Read the model definition and answer for the solid it produces. Units are mm, in the model's axes. A direction names the side the tool comes from. Coordinates: 2 decimals unless noted, no trailing zeros. Write each loop counter-clockwise with the first axis right and the second up, starting at its lowest first coordinate (ties: lowest second). Pieces come first, ordered by that corner, then holes.
Item 1: Section D-D (x = 66.04) is taken. Give the vertices of the cut face in (y, z), then the cut area to 3 significant figures.
Item 2: Section C-C (y = 1.5) is taken. State how many separate pieces and enclosed holes the cut face has, then the cut area to 3 significant figures.
Item 3: Section A-A (z = 0) is taken. Give the vertices of the cut face in (x, y) (3 decimals), then the cut area to 3 significant figures.
Item 4: Determine the mould class of faces 3 (the face through (-46.367, 3.131, -60.47)), 4 (the face through (1, 0, 33)), 5 (the face through (69.262, 3.219, 1.015)) for opening direction X: released by +X, released by -X, zero draft, split by the parting line, or undercut.
Item 5: Section B-B (x = 0) is taken. Give the vertices of the cut face in (y, z) (3 decimals).
Item 6: Straight lines are drawn through the part: probe 1 along X at (y, z) = (1, -0.5); probe 2 along X at (y, z) = (2.25, 3); probe 3 along Z at (x, y) = (46, 3.75). For each, find the intervals that lie inside material, in ascending order.
Item 7: Each of these flat-tipped pins is pushed along its axis until it touches: P1, Ø11, axis at x = 46.7, z = 46.7, coming from the +Y side; P2, Ø5.5, axis at x = 46.7, z = -46.7, coming from the -Y side; P3, Ø3, axis at x = -43.5, y = 3, coming from the +Z side; P4, Ø2, axis at y = 4, z = 37, coming from the -X side. Where does it stop, or does it pass through?
Item 8: A tool of negligible diameter and unlimited length cuts with its end or side. For faces 1 (the face through (48.755, 3.219, -44.018)), 2 (the face through (-34.094, 4.114, -7.571)), from which of +Z, -Z, +X, -X, +Y, -Y can it reach the whole face along a straight path? Write none if from no direction.
from build123d import *

# Parameters (mm, degrees)
SKETCH1_R           = 76.2
SKETCH1_R_2         = 34.925
BOSS_EXTRUDE1_DEPTH = 6.35
CIRPATTERN1_COUNT   = 8
CHAMFER1_SIZE       = 1.27
SKETCH6_R           = 34.925
SKETCH6_R_2         = 31.75
BOSS_EXTRUDE2_DEPTH = 3.175


with BuildPart() as part:
    # Sketch1 → Boss-Extrude1 (new body)
    with BuildSketch(Plane(origin=(0, 0, 0), x_dir=(1, 0, 0), z_dir=(0, 1, 0))):
        with Locations(Location((0, 0, 0), (0, 0, 270))):
            Circle(SKETCH1_R)
        with Locations(Location((0, 0, 0), (0, 0, 270))):
            Circle(SKETCH1_R_2, mode=Mode.SUBTRACT)
    extrude(amount=BOSS_EXTRUDE1_DEPTH)

    # Sketch4 → 1_4 Clearance Hole1 (revolve, cut)
    with BuildSketch(Plane(origin=(0, 6.35, 66.04), x_dir=(0, 0, 1), z_dir=(1, 0, 0))):
        Polygon((0, 0), (0, 27.429827343), (3.3782, 25.4), (3.3782, 0), align=None)
    f_1_4_clearance_hole1 = revolve(axis=Axis((0, 12.7, 66.04), (0, -1, 0)), mode=Mode.SUBTRACT)

    # CirPattern1: 1_4 Clearance Hole1 ×8 about axis
    cirpattern1_axis = Axis((0, 0, 0), (0, 1, 0))
    for i in range(1, CIRPATTERN1_COUNT):
        add(f_1_4_clearance_hole1.rotate(cirpattern1_axis, i * 360 / CIRPATTERN1_COUNT), mode=Mode.SUBTRACT)

    # Chamfer1
    chamfer1_edges = [part.edges().sort_by_distance(p)[0] for p in [
        (0, 6.35, -34.925),
    ]]
    chamfer(chamfer1_edges, length=CHAMFER1_SIZE)

    # Sketch6 → Boss-Extrude2 (add)
    with BuildSketch(Plane(origin=(0, 0, 0), x_dir=(1, 0, 0), z_dir=(0, 1, 0))):
        with Locations(Location((0, 0, 0), (0, 0, 270))):
            Circle(SKETCH6_R)
        with Locations(Location((0, 0, 0), (0, 0, 270))):
            Circle(SKETCH6_R_2, mode=Mode.SUBTRACT)
    extrude(amount=BOSS_EXTRUDE2_DEPTH)


solid = part.part
Established:
1. outline: (0, -38.02) - (6.35, -38.02) - (6.35, -3.38) - (0, -3.38) - close; (0, 3.38) - (6.35, 3.38) - (6.35, 38.02) - (0, 38.02) - close
1. area: 440 mm2
2. separate pieces: 1
2. enclosed holes: 9
2. area: 14,800 mm2
3. outline: (-76.2, 0) - (-69.418, 0) - (-69.418, 6.35) - (-76.2, 6.35) - close; (-62.662, 0) - (-31.75, 0) - (-31.75, 3.175) - (-34.925, 3.175) - (-34.925, 5.08) - (-36.195, 6.35) - (-62.662, 6.35) - close; (31.75, 0) - (62.662, 0) - (62.662, 6.35) - (36.195, 6.35) - (34.925, 5.08) - (34.925, 3.175) - (31.75, 3.175) - close; (69.418, 0) - (76.2, 0) - (76.2, 6.35) - (69.418, 6.35) - close
3. area: 457 mm2
4. face 3: split by the parting line
4. face 4: zero draft
4. face 5: undercut
5. outline: (0, -76.2) - (6.35, -76.2) - (6.35, -69.418) - (0, -69.418) - close; (0, -62.662) - (6.35, -62.662) - (6.35, -36.195) - (5.08, -34.925) - (3.175, -34.925) - (3.175, -31.75) - (0, -31.75) - close; (0, 31.75) - (3.175, 31.75) - (3.175, 34.925) - (5.08, 34.925) - (6.35, 36.195) - (6.35, 62.662) - (0, 62.662) - close; (0, 69.418) - (6.35, 69.418) - (6.35, 76.2) - (0, 76.2) - close
6. probe 1: x = -76.2 to -69.38, -62.7 to -31.75, 31.75 to 62.7, 69.38 to 76.2
6. probe 2: x = -76.14 to -67.59, -64.49 to -31.61, 31.61 to 64.49, 67.59 to 76.14
6. probe 3: z = -60.75 to -50, -43.39 to 43.39, 50 to 60.75
7. P1: stops at y = 6.35
7. P2: passes through
7. P3: stops at z = 63.58
7. P4: stops at x = -67.16
8. face 1: +Y, -Y
8. face 2: +Y
